CAD build for the part. Positions are in the model's coordinates, mm. A direction names the side the tool comes from. Coordinates: 2 decimals unless noted, no trailing zeros. Loops run counter-clockwise (first coordinate to the right, second up) from the corner with the lowest first, then second, coordinate; pieces in that order, holes last. Notation, with made-up numbers: (49.5, -2.75) -> (87.5, -2.75) arc R7 cw to (87.5, 3.25) -> close; hole circle Ø6 at (-15, -36). An arc over 180 degrees is marked (long way). Write each question's results on one line, items separated by ' | '.
from build123d import *

# Parameters (mm, degrees)
BOSS_EXTRUDE1_DEPTH = 15
CUT_EXTRUDE1_REACH  = 143.188
SKETCH2_R           = 3
SKETCH3_R           = 4.25
CUT_EXTRUDE2_DEPTH  = 30
FILLET3_R           = 7
CHAMFER1_SIZE       = 10
CHAMFER1_SIZE2      = 17.320508076
FILLET4_R           = 2


with BuildPart() as part:
    # Sketch1 → Boss-Extrude1 (new, symmetric)
    with BuildSketch(Plane.XY):
        Polygon((0, 0), (0, 27), (-3, 27), (-3, 53), (-130, 53), (-130, 35), (-18, 35), (-18, 0), align=None)
    extrude(amount=BOSS_EXTRUDE1_DEPTH, both=True)

    # Sketch2 → Cut-Extrude1 (cut, up to next)
    with BuildSketch(Plane(origin=(0, 0, 0), x_dir=(0, 0, -1), z_dir=(1, 0, 0)), mode=Mode.PRIVATE) as cut_extrude1_sk1:
        with Locations((0, 22)):
            Circle(SKETCH2_R)
    cut_extrude1_tool1 = extrude(cut_extrude1_sk1.sketch, amount=-CUT_EXTRUDE1_REACH, mode=Mode.PRIVATE) & part.part
    # Sketch2 → Cut-Extrude1 (cut, up to next)
    with BuildSketch(Plane(origin=(0, 0, 0), x_dir=(0, 0, -1), z_dir=(1, 0, 0)), mode=Mode.PRIVATE) as cut_extrude1_sk2:
        with BuildLine():
            Line((3, 12), (3, 7))
            ThreePointArc((3, 7), (0, 4), (-3, 7))
            Line((-3, 7), (-3, 12))
            ThreePointArc((-3, 12), (0, 15), (3, 12))
        make_face()
    cut_extrude1_tool2 = extrude(cut_extrude1_sk2.sketch, amount=-CUT_EXTRUDE1_REACH, mode=Mode.PRIVATE) & part.part
    add(cut_extrude1_tool1.solids().sort_by_distance((0, 22, 0))[0], mode=Mode.SUBTRACT)
    add(cut_extrude1_tool2.solids().sort_by_distance((0, 9.5, 0))[0], mode=Mode.SUBTRACT)

    # Sketch3 → Cut-Extrude2 (cut)
    with BuildSketch(Plane.XZ.offset(-35)):
        with Locations(Location((-110, 0, 0), (0, 0, 270))):
            Circle(SKETCH3_R)
        with Locations(Location((-70, 0, 0), (0, 0, 270))):
            Circle(SKETCH3_R)
    extrude(amount=-CUT_EXTRUDE2_DEPTH, mode=Mode.SUBTRACT)

    # Fillet3
    fillet3_edges = [part.edges().sort_by_distance(p)[0] for p in [
        (-18, 35, 0),
    ]]
    fillet(fillet3_edges, radius=FILLET3_R)

    # Chamfer1
    chamfer1_edges = [part.edges().sort_by_distance(p)[0] for p in [
        (-3, 53, 0),
    ]]
    chamfer1_side = [part.faces().sort_by_distance(p)[0] for p in [
        (-3, 40, 0),
    ]]
    chamfer(chamfer1_edges, length=CHAMFER1_SIZE, length2=CHAMFER1_SIZE2, reference=chamfer1_side[0])

    # Fillet4
    fillet4_edges = [part.edges().sort_by_distance(p)[0] for p in [
        (-3, 27, 0),
    ]]
    fillet(fillet4_edges, radius=FILLET4_R)


solid = part.part
1) Slice it at C-C (z = -10.25). Write the cut outline in (x, y), then the cut area to 3 significant figures.
Outcome:
outline: (-130, 35) -> (-25, 35) arc R7 cw to (-18, 28) -> (-18, 0) -> (0, 0) -> (0, 27) -> (-1, 27) arc R2 cw to (-3, 29) -> (-3, 43) -> (-20.32, 53) -> (-130, 53) -> close | area: 2,820 mm^2
2) Slice it at B-B (y = 22). Write the cut outline in (x, z), then the cut area to 3 significant figures.
Outcome:
outline: (-18, -15) -> (0, -15) -> (0, -3) -> (-18, -3) -> close; (-18, 3) -> (0, 3) -> (0, 15) -> (-18, 15) -> close | area: 432 mm^2
3) Two-plate mould, pull along Z, no slides. Class faces 5 (the flat face through (-51, 39, -15)), 6 (the cylindrical face through (-8.87, 19.07, 0.65)), 7 (the flat face through (-18, 17, 0)): pulls with the +Z half, pulls with the -Z half, needs draft (parallel to the pull), parting line crosses it, or undercut.
Outcome:
face 5: pulls with the -Z half | face 6: undercut | face 7: needs draft
4) Which spindle directions (+Z, -Z, +X, -X, +Y, -Y) get a long thin tool onto all of the face, cutting with end or side? Do faces 1 (the cylindrical face through (-9, 4, 0)), 2 (the cylindrical face through (-106.416, 43.874, -2.285)), 3 (the flat face through (-3, 36, 0)), 4 (the flat face through (-78, 35, 0)). Say none if no direction does.
Outcome:
face 1: +X, -X | face 2: +Y, -Y | face 3: +Z, -Z, +X, +Y | face 4: +Z, -Z, -X, -Y
5) Slice it at D-D (y = 46). Write the cut outline in (x, z).
Outcome:
outline: (-130, -15) -> (-8.2, -15) -> (-8.2, 15) -> (-130, 15) -> close; hole circle Ø8.5 at (-110, 0); hole circle Ø8.5 at (-70, 0)
6) Pin check, flat tips, straight feed: pin 1 (5 mm diameter, centred on x = -21, y = 13, fed in from +Z); pin 2 (7 mm diameter, centred on y = 33, z = 3, fed in from +X); pin 3 (14 mm diameter, centred on y = 8, z = -7, fed in from -X); pin 4 (1 mm diameter, centred on x = -105.5, z = -10, fed in from -Y). Stop position of each tip, or through.
Outcome:
pin 1: passes through | pin 2: stops at x = -3 | pin 3: stops at x = -18 | pin 4: stops at y = 35
7) Slice it at A-A (x = -110). Write the cut outline in (y, z), then the cut area to 3 significant figures.
Outcome:
outline: (35, -15) -> (53, -15) -> (53, -4.25) -> (35, -4.25) -> close; (35, 4.25) -> (53, 4.25) -> (53, 15) -> (35, 15) -> close | area: 387 mm^2
8) Drill centre lines: L1, parallel to X at y = 40.25, z = 0; L2, parallel to Y at x = -13.25, z = 0; L3, parallel to X at y = 4, z = 6.75. Where is each one in solid material? Low to high. Write a range as from..to.
Outcome:
L1: x = -130..-114.25, -105.75..-74.25, -65.75..-3 | L2: y = 0..4, 15..19, 25..48.92 | L3: x = -18..0
